Autodesk Inventor part; units mm, degrees
ref_plane "YZ Plane" through (0, 0, 0) normal (1, 0, 0) x (0, 1, 0)
ref_plane "XZ Plane" through (0, 0, 0) normal (0, 1, 0) x (-1, 0, 0)
ref_plane "XY Plane" through (0, 0, 0) normal (0, 0, 1) x (1, 0, 0)
sketch "Sketch1" plane through (0, 0, 0) normal (0, 1, 0) x (-1, 0, 0)
  circle A0 centre (0, 0) radius 8.0947
  circle A1 centre (23.57, 23.57) radius 2.6
  circle A2 centre (23.57, -23.57) radius 2.6
  circle A3 centre (-23.57, -23.57) radius 2.6
  circle A4 centre (-23.57, 23.57) radius 2.6
  circle A5 centre (23.57, 23.57) radius 7.3625 construction
  circle A6 centre (23.57, -23.57) radius 7.3625 construction
  circle A7 centre (-23.57, -23.57) radius 7.3625 construction
  circle A8 centre (-23.57, 23.57) radius 7.3625 construction
  line L0 (23.57, 30.9325) -> (-23.57, 30.9325)
  line L1 (-30.9325, 23.57) -> (-30.9325, -23.57)
  line L2 (-23.57, -30.9325) -> (23.57, -30.9325)
  arc A9 (18.3639, 18.3639) -> (23.57, 30.9325) centre (23.57, 23.57) ccw
  arc A10 (23.57, -30.9325) -> (18.3639, -18.3639) centre (23.57, -23.57) ccw
  circle A11 centre (0, 0) radius 25.9705 construction
  arc A12 (18.3639, 18.3639) -> (18.3639, -18.3639) centre (0, 0) ccw
  arc A13 (-23.57, 30.9325) -> (-30.9325, 23.57) centre (-23.57, 23.57) ccw
  arc A14 (-30.9325, -23.57) -> (-23.57, -30.9325) centre (-23.57, -23.57) ccw
  dimension "d0" = 16.1894
  dimension "d1" = 5.2
  dimension "d2" = 23.57
  dimension "d3" = 23.57
  dimension "d4" = 23.57
  dimension "d5" = 23.57
  dimension "d6" = 4.7625
extrude "Extrusion1" add sketch "Sketch1" along normal blind 31.2375 contours A9 A12 A10 L2 A14 L1 A13 L0
properties part number "CNC-009-XAxisNema23Spacer" material "ABS Plastic"
The listing builds one solid part. Answer for the finished solid, in the listing's coordinates (mm). Coordinates: 2 decimals unless noted, no trailing zeros. Write each loop counter-clockwise with the first axis right and the second up, starting at its lowest first coordinate (ties: lowest second). Pieces come first, ordered by that corner, then holes. Notation, with made-up numbers: M 63,39.25 L 103,39.25 A20 cw 103,78.25 Z; hole C 31.5,-29.75 d1. An arc over 180 degrees is marked long. Use one line per item in the form item = value.
Item 1: Find section A-A, the plane x = 0. Give the vertices of the cut face in (y, z), plus the area to 3 significant figures.
Model answer:
outline = M 0,-30.93 L 31.24,-30.93 L 31.24,-25.97 L 0,-25.97 Z; M 0,25.97 L 31.24,25.97 L 31.24,30.93 L 0,30.93 Z
area = 310 mm2
Item 2: Find section B-B, the plane y = 26.5. Give the vertices of the cut face in (x, z) (1 decimal), plus the area to 3 significant figures.
Model answer:
outline = M -23.6,-30.9 L 23.6,-30.9 A7.4 ccw 30.9,-23.6 L 30.9,23.6 A7.4 ccw 23.6,30.9 L -23.6,30.9 A7.4 ccw long -18.4,18.4 A26 cw long -18.4,-18.4 A7.4 ccw long Z; hole C -23.6,-23.6 d5.2; hole C -23.6,23.6 d5.2; hole C 23.6,-23.6 d5.2; hole C 23.6,23.6 d5.2
area = 1,330 mm2
Item 3: The mould has two halves that part along Z. Classify faces 1 (the face through (0, 15, -30.932)), 2 (the face through (28, 31.238, 0)), 3 (the face through (-30.292, 15.4, -20.567)): released by +Z, released by -Z, zero draft, split by the parting line, or undercut.
Model answer:
face_1 = released by -Z
face_2 = zero draft
face_3 = undercut
Item 4: Find section C-C, the plane z = 17. Give the vertices of the cut face in (x, y), plus the area to 3 significant figures.
Model answer:
outline = M -26.89,0 L -20.25,0 L -20.25,31.24 L -26.89,31.24 Z; M 19.63,0 L 30.93,0 L 30.93,31.24 L 19.63,31.24 Z
area = 561 mm2
Item 5: Find the intervals of material crossed by probe 1 along Z at (x, y) = (-23.57, 8); probe 2 along Z at (x, y) = (-23, 22); probe 3 along Z at (x, y) = (0, 25.5), in increasing order.
Model answer:
probe_1 = -30.93 to -26.17, -20.97 to -16.21, 16.21 to 20.97, 26.17 to 30.93
probe_2 = -30.93 to -26.11, -21.03 to -16.23, 16.23 to 21.03, 26.11 to 30.93
probe_3 = -30.93 to -25.97, 25.97 to 30.93
Item 6: Given P1, Ø2, axis at y = 10, z = 6.5, coming from the -X side; P2, Ø3, axis at x = 23.57, z = -23.57, coming from the -Y side, each flat-ended and moving along its own axis, determine where each tip first touches the part or whether it passes through.
Model answer:
P1 = 24.86
P2 = through
Item 7: Find section D-D, the plane x = -24.5. Give the vertices of the cut face in (y, z).
Model answer:
outline = M 0,-30.87 L 31.24,-30.87 L 31.24,-26 L 0,-26 Z; M 0,-21.14 L 31.24,-21.14 L 31.24,-16.27 L 0,-16.27 Z; M 0,16.27 L 31.24,16.27 L 31.24,21.14 L 0,21.14 Z; M 0,26 L 31.24,26 L 31.24,30.87 L 0,30.87 Z
